```python
from build123d import *

# Parameters (mm, degrees)
F0_R     = 19.05
F0_R_2   = 7.5
F1_DEPTH = 30
F2_R     = 29.05
F2_R_2   = 7.5
F3_DEPTH = 5
F4_R     = 12.5
F4_R_2   = 7.5
F5_DEPTH = 15
F6_SIZE  = 1
F7_R     = 2.5
F8_DEPTH = 25


with BuildPart() as f1:
    # F0 (on Right) → F1 (new body, symmetric)
    with BuildSketch(Plane.YZ):
        Circle(F0_R)
        Circle(F0_R_2, mode=Mode.SUBTRACT)
    extrude(amount=F1_DEPTH, both=True)

    # F2 (on face) → F3 (join)
    with BuildSketch(Plane.YZ.offset(30)):
        Circle(F2_R)
        Circle(F2_R_2, mode=Mode.SUBTRACT)
    extrude(amount=F3_DEPTH)

    # F4 (on face) → F5 (join)
    with BuildSketch(Plane.YZ.offset(35)):
        Circle(F4_R)
        Circle(F4_R_2, mode=Mode.SUBTRACT)
    extrude(amount=F5_DEPTH)

    # F6
    f6_edges = [f1.edges().sort_by_distance(p)[0] for p in [
        (35, -29.05, 0),
        (30, -29.05, 0),
        (50, -12.5, 0),
        (50, -7.5, 0),
    ]]
    chamfer(f6_edges, length=F6_SIZE)

    # F7 (on Top) → F8 (cut, symmetric)
    with BuildSketch(Plane.XY):
        with Locations((42.5, 0)):
            Circle(F7_R)
    extrude(amount=F8_DEPTH, both=True, mode=Mode.SUBTRACT)

    # F9: F1 across plane


with BuildPart() as f1_1:
    add(f1.part)
    add(f1.part.mirror(Plane.YZ))


solid = f1_1.part
```
Model file for the job. Use its own axes, mm. A direction names the side the tool comes from. Coordinates: 2 decimals unless noted, no trailing zeros. Order: outer loops, then holes, each group sorted by start corner. A loop starts at its lowest first (then second) coordinate and runs counter-clockwise, first axis right, second up. Notation, with made-up numbers: (-16.5, 20) -> (25.5, 20) arc R26 cw to (25.5, 46) -> close; hole circle Ø5 at (40, -24.75). An arc over 180 degrees is marked (long way). Answer as a JSON object with one key per item and string values. Group by question number.
1) Drill centre lines: L1, parallel to X at y = 0, z = -9; L2, parallel to X at y = 19, z = 6; L3, parallel to Z at x = -37.25, y = 0. Where is each one in solid material? Low to high.
2) Cut at B-B, the plane x = 21.5. Write the cut outline in (y, z), then the cut area to 3 significant figures.
3) Which spindle directions (+Z, -Z, +X, -X, +Y, -Y) get a long thin tool onto all of the face, cutting with end or side? Do faces 1 (the face through (35, 6, -12)), 2 (the face through (-41.9, 5.77, -11.09)), 3 (the face through (0.42, -15.12, -11.59)). Say none if no direction does.
4) Cut at A-A, the plane x = -42.5. Write the cut outline in (y, z).
5) Pull direction X, two halves, no side cores. Call faces 4 (the face through (50, -4, -8)), 5 (the face through (-35, 6, -12)), 6 (the face through (42.17, 2.48, -9.75)): +X half, -X half, draft (parallel to the pull), parting line (faces both ways), or undercut.
6) Flat gauge pins, fed straight in: pin 1 (6 mm diameter, centred on y = -9, z = -13.5, fed in from +X); pin 2 (8 mm diameter, centred on x = 14, y = 12.5, fed in from +Z); pin 3 (3 mm diameter, centred on x = 26, z = -10.5, fed in from +Y). Where does each tip first touch, or does it go through?
Check values:
{
 "1": {"L1": "x = -50 to -45, -40 to 40, 45 to 50", "L2": "x = -35 to -30, 30 to 35", "L3": "z = -12.5 to -7.5, 7.5 to 12.5"},
 "2": {"outline": "circle Ø38.1 at (0, 0); hole circle Ø15 at (0, 0)", "area": "963 mm²"},
 "3": {"face 1": "+X", "face 2": "-X", "face 3": "none"},
 "4": {"outline": "(-2.5, -12.25) -> (-2.5, -7.07) arc R7.5 cw to (-2.5, 7.07) -> (-2.5, 12.25) arc R12.5 ccw to start; (2.5, -12.25) arc R12.5 ccw to (2.5, 12.25) -> (2.5, 7.07) arc R7.5 cw to (2.5, -7.07) -> close"},
 "5": {"face 4": "+X half", "face 5": "-X half", "face 6": "undercut"},
 "6": {"pin 1": "stops at x = 35", "pin 2": "stops at z = 17.05", "pin 3": "stops at y = 16.79"}
}
